Read the model definition and answer for the solid it produces. Units are mm, in the model's axes. A direction names the side the tool comes from. Coordinates: 2 decimals unless noted, no trailing zeros. Write each loop counter-clockwise with the first axis right and the second up, starting at its lowest first coordinate (ties: lowest second). Pieces come first, ordered by that corner, then holes. Notation, with made-up numbers: (55.5, 40.25) - (86.5, 40.25) arc R23 ccw to (86.5, 58.25) - close; hole circle Ø7 at (86.5, 70). An arc over 180 degrees is marked (long way). Return JSON: item names as keys, results as strings.
```python
from build123d import *

# Parameters (mm, degrees)
EXTRUDE_THIN1_DEPTH        = 43
SKETCH7_W                  = 27
SKETCH7_H                  = 15
CUT_EXTRUDE3_DEPTH         = 15
FILLET1_R                  = 6.35
SKETCH11_W                 = 17
SKETCH11_H                 = 86
BOSS_EXTRUDE1_DEPTH        = 3
F_10_24_TAPPED_HOLE2_D     = 3.7973
FILLET2_R                  = 6.35
F_10_CLEARANCE_HOLE2_D     = 5.6134
F_10_CLEARANCE_HOLE2_DEPTH = 9.53
F_10_CLEARANCE_HOLE2_TIP   = 1.686435499


with BuildPart() as part:
    # Sketch1 → Extrude-Thin1 (new body, symmetric)
    with BuildSketch(Plane(origin=(0, 0, 0), x_dir=(1, 0, 0), z_dir=(0, 1, 0))):
        Polygon((0, 0), (0, 17), (-15, 17), (-15, 44), (-32, 44), (-32, 41), (-18, 41), (-18, 14), (-3, 14), (-3, 0), align=None)
    extrude(amount=EXTRUDE_THIN1_DEPTH, both=True)

    # Sketch7 → Cut-Extrude3 (cut)
    with BuildSketch(Plane.ZY.offset(18)):
        with Locations((-27.5, 35.5)):
            Rectangle(SKETCH7_W, SKETCH7_H)
    cut_extrude3 = extrude(amount=-CUT_EXTRUDE3_DEPTH, mode=Mode.SUBTRACT)

    # Mirror3: Cut-Extrude3 across plane
    add(cut_extrude3.mirror(Plane.ZX), mode=Mode.SUBTRACT)

    # Fillet1
    fillet1_edges = [part.edges().sort_by_distance(p)[0] for p in [
        (-16.5, 28, -41),
        (-16.5, -28, -41),
    ]]
    fillet(fillet1_edges, radius=FILLET1_R)

    # Sketch11 → Boss-Extrude1 (add)
    with BuildSketch(Plane(origin=(0, 0, -44), x_dir=(-1, 0, 0), z_dir=(0, 0, -1))):
        with Locations((23.5, 0)):
            Rectangle(SKETCH11_W, SKETCH11_H)
    extrude(amount=BOSS_EXTRUDE1_DEPTH)

    # #10-24 Tapped Hole2 (through all)
    with Locations(Plane(origin=(-13.4585207, 10.001554842, -47), x_dir=(-1, 0, 0), z_dir=(0, 0, -1))):
        with Locations((7.0414793, -27.001554842), (7.0414793, 24.998445158), (7.0414793, 6.998445158), (7.0414793, -45.001554842)):
            Hole(F_10_24_TAPPED_HOLE2_D / 2)

    # Fillet2
    fillet2_edges = [part.edges().sort_by_distance(p)[0] for p in [
        (-32, -43, -44),
        (-32, 43, -44),
    ]]
    fillet(fillet2_edges, radius=FILLET2_R)

    # #10 Clearance Hole2
    with Locations(Plane.ZY.offset(3)):
        with Locations((-7, -35), (-7, 35)):
            Hole(F_10_CLEARANCE_HOLE2_D / 2, depth=F_10_CLEARANCE_HOLE2_DEPTH)
            with Locations((0, 0, -(F_10_CLEARANCE_HOLE2_DEPTH + F_10_CLEARANCE_HOLE2_TIP / 2))):  # 118° drill point
                Cone(0, F_10_CLEARANCE_HOLE2_D / 2, F_10_CLEARANCE_HOLE2_TIP, mode=Mode.SUBTRACT)


solid = part.part
```
(1) Determine the mould class of faces 3 (the face through (-26, 1, -41)), 4 (the face through (-19.48, -15.4, -43.96)), 5 (the face through (-15, -1, -35)) for opening direction X: +X half, -X half, draft (parallel to the pull), parting line (faces both ways), or undercut.
Answer:
{"face 3": "draft", "face 4": "undercut", "face 5": "+X half"}
(2) A cutting plane is placed at C-C (z = -7). Determine the outline of the cut face in (x, y).
Answer:
{"outline": "(-3, -43) - (0, -43) - (0, -37.81) - (-3, -37.81) - close; (-3, -32.19) - (0, -32.19) - (0, 32.19) - (-3, 32.19) - close; (-3, 37.81) - (0, 37.81) - (0, 43) - (-3, 43) - close"}
(3) A cutting plane is placed at A-A (y = -17). Determine the outline of the cut face in (x, z).
Answer:
{"outline": "(-32, -47) - (-22.4, -47) - (-22.4, -41) - (-32, -41) - close; (-18.6, -47) - (-15, -47) - (-15, -17) - (0, -17) - (0, 0) - (-3, 0) - (-3, -14) - (-18, -14) - (-18, -41) - (-18.6, -41) - close"}
(4) Which of the six approach directions +Z, -Z, +X, -X, +Y, -Y give full straight-line access (tool end or side, diameter ignored) to faces 1 (the face through (-11, 0, -14)), 2 (the face through (-30.09, -41.19, -44.04))?
Answer:
{"face 1": "+Z, -X, +Y, -Y", "face 2": "+Z, -Z, -X, -Y"}
(5) Straight lines are drawn through the part: line 1 (Y direction, x = -20.5, z = -45.2); line 2 (Y direction, x = -2.4, z = -7); line 3 (Y direction, x = -20, z = -43). For each, find the intervals that lie inside material, in ascending order. Write a range as from..to.
Answer:
{"line 1": "-43..-36.9, -33.1..-18.9, -15.1..15.1, 18.9..33.1, 36.9..43", "line 2": "-43..-37.81, -32.19..32.19, 37.81..43", "line 3": "-43..-36.83, -33.17..-18.83, -15.17..15.17, 18.83..33.17, 36.83..43"}
(6) A cutting plane is placed at B-B (x = -20.5). Determine the outline of the cut face in (y, z).
Answer:
{"outline": "(-43, -47) - (-36.9, -47) - (-36.9, -41) - (-43, -41) - close; (-33.1, -47) - (-18.9, -47) - (-18.9, -41) - (-33.1, -41) - close; (-15.1, -47) - (15.1, -47) - (15.1, -41) - (-15.1, -41) - close; (18.9, -47) - (33.1, -47) - (33.1, -41) - (18.9, -41) - close; (36.9, -47) - (43, -47) - (43, -41) - (36.9, -41) - close"}
(7) Flat-ended cylindrical pins translate along their axes: P1, Ø1.5, axis at y = -29, z = -24, coming from the +X side; P2, Ø8, axis at x = -14, z = -34.5, coming from the -Y side; P3, Ø18.5, axis at y = -10.5, z = -8, coming from the -X side; P4, Ø5, axis at x = -15.5, z = -22, coming from the -Y side. Find the tip coordinate at first contact, or state that the pin passes through.
Answer:
{"P1": "through", "P2": "y = -29.21", "P3": "x = -18", "P4": "y = -28"}
(8) A cutting plane is placed at D-D (y = -5). Determine the outline of the cut face in (x, z).
Answer:
{"outline": "(-32, -47) - (-15, -47) - (-15, -17) - (0, -17) - (0, 0) - (-3, 0) - (-3, -14) - (-18, -14) - (-18, -41) - (-32, -41) - close"}
